```python
from build123d import *

# Parameters (mm, degrees)
F0_W     = 35
F0_H     = 25
F1_DEPTH = 400
F3_DEPTH = 25
F5_DEPTH = 10


with BuildPart() as f1:
    # F0 (on Top) → F1 (new body)
    with BuildSketch(Plane.XY):
        with Locations((-42.358379, -48.249161)):
            Rectangle(F0_W, F0_H)
    extrude(amount=F1_DEPTH)

    # F2 (on face) → F3 (join)
    with BuildSketch(Plane(origin=(0, 0, 0), x_dir=(1, 0, 0), z_dir=(0, 0, -1))):
        Polygon((-49.858379, 35.749161), (-24.858379, 60.749161), (-59.858379, 60.749161), (-59.858379, 35.749161), align=None)
    extrude(amount=F3_DEPTH)

    # F4 (on face) → F5 (join)
    with BuildSketch(Plane(origin=(0, 0, -25), x_dir=(1, 0, 0), z_dir=(0, 0, -1))):
        Polygon((-24.858379, 60.749161), (-59.858379, 60.749161), (-59.858379, 35.749161), (-49.858379, 35.749161), align=None)
        Polygon((-24.858379, 35.749161), (-24.858379, 60.749161), (-49.858379, 35.749161), align=None)
    extrude(amount=F5_DEPTH)


solid = f1.part
```
The listing builds one solid part. Answer for the finished solid, in the listing's coordinates (mm). A direction names the side the tool comes from. Round coordinates to 2 decimals unless told otherwise and drop trailing zeros. Order: outer loops, then holes, each group sorted by start corner. A loop starts at its lowest first (then second) coordinate and runs counter-clockwise, first axis right, second up. Notation, with made-up numbers: (-39, 69.25) - (0, 69.25) arc R33 ccw to (0, 106.25) - close; hole circle Ø10 at (82.25, 2.25). An arc over 180 degrees is marked (long way). Put each result on its own line as item: value. Start each with the question number.
(1) Determine the mould class of faces 1 (the flat face through (-24.858, -48, 197)), 2 (the flat face through (-43, -48, 400)), 3 (the flat face through (-37.533, -48.074, -12.325)) for opening direction Z: released by +Z, released by -Z, zero draft, split by the parting line, or undercut.
(2) For faces 4 (the flat face through (-24.858, -48, -30)), 5 (the flat face through (-32, -43, -25)), determine the directions among +Z, -Z, +X, -X, +Y, -Y from which every point of the face is accessible in a straight line to the end or side of a thin tool.
(3) Find section A-A (y = -51.5). Give the vertices of the cut face in (x, z), plus the area to 3 significant figures.
(4) A straight line is drawn through the part: probe 1 along Z at (x, y) = (-33.5, -48.5). Find the intervals that lie inside material, in ascending order. Write a range as from..to.
(5) Find section B-B (z = -8). Give the vertices of the cut face in (x, y), plus the area to 4 significant figures.
Reply:
1. face 1: zero draft
1. face 2: released by +Z
1. face 3: undercut
2. face 4: +Z, -Z, +X, +Y, -Y
2. face 5: +X, +Y
3. outline: (-59.86, -35) - (-24.86, -35) - (-24.86, -25) - (-34.11, -25) - (-34.11, 0) - (-24.86, 0) - (-24.86, 400) - (-59.86, 400) - close
3. area: 15,000 mm^2
4. probe 1: -35..-25, 0..400
5. outline: (-59.86, -60.75) - (-24.86, -60.75) - (-49.86, -35.75) - (-59.86, -35.75) - close
5. area: 562.5 mm^2
